The figure shows three views and two pictorial views of one solid part (mm, origin at its lowest corner). Answer the questions. A direction names the side the tool comes from. Coordinates: 2 decimals unless noted, no trailing zeros. Write each loop counter-clockwise with the first axis right and the second up, starting at its lowest first coordinate (ties: lowest second). Pieces come first, ordered by that corner, then holes. Notation, with made-up numbers: M 8.5,-3.5 L 18.5,-3.5 A7 cw 18.5,8.5 Z; hole C 79.5,72 d10. An arc over 180 degrees is marked long. Answer as CSV lines item,"result".
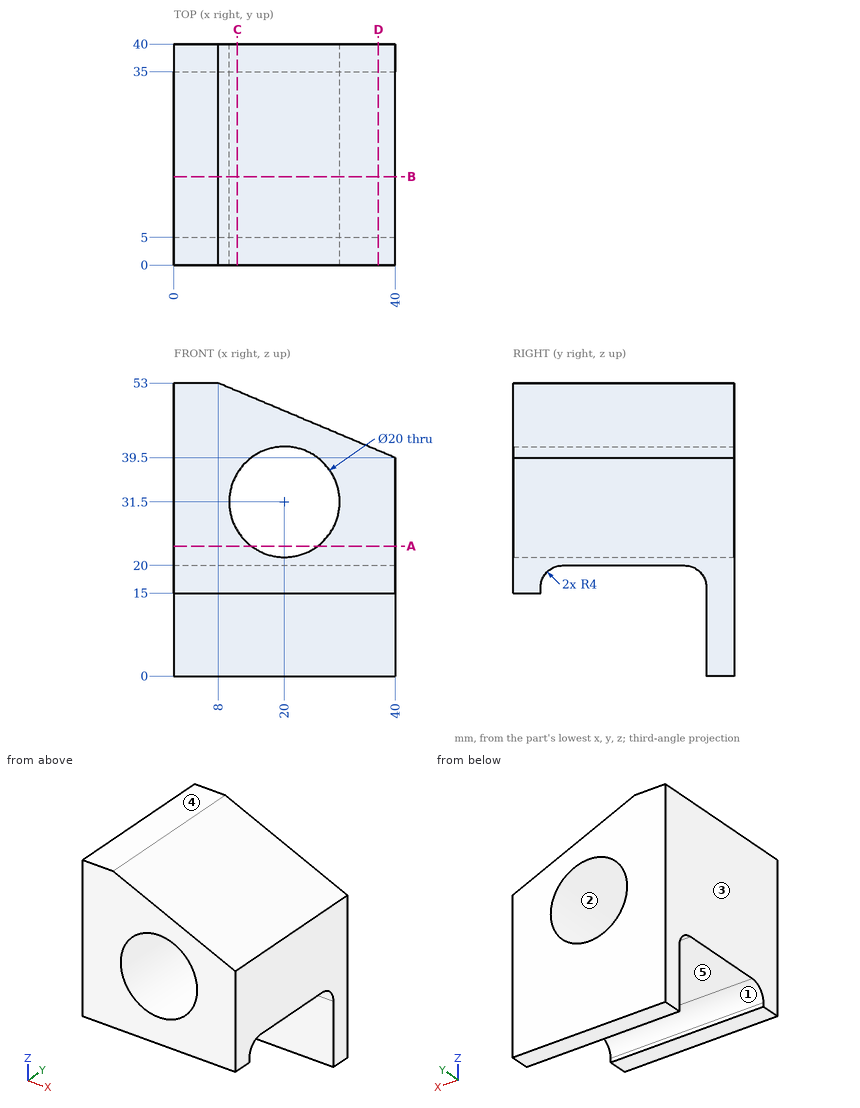
Q1. Flat-ended cylindrical pins translate along their axes: pin 1 Ø6 at (x, y) = (32, 19.5) entering from -Z; pin 2 Ø2.5 at (x, y) = (19, 3) entering from -Z; pin 3 Ø24 at (x, y) = (16.5, 21.5) entering from -Z. Find the tip coordinate at first contact, or state that the pin passes through.
Output:
pin 1,"z = 20"
pin 2,"z = 15"
pin 3,"z = 19.12"
Q2. Find section A-A (z = 23.5). Give the vertices of the cut face in (x, y).
Output:
outline,"M 0,0 L 14,0 L 14,40 L 0,40 Z; M 26,0 L 40,0 L 40,40 L 26,40 Z"
Q3. Find section D-D (x = 37). Give the vertices of the cut face in (y, z).
Output:
outline,"M 0,15 L 5,15 L 5,16 A4 cw 9,20 L 31,20 A4 cw 35,16 L 35,0 L 40,0 L 40,40.77 L 0,40.77 Z"
Q4. Find section B-B (y = 16). Give the vertices of the cut face in (x, z), and give its area (3 significant figures).
Output:
outline,"M 0,20 L 40,20 L 40,39.5 L 8,53 L 0,53 Z; hole C 20,31.5 d20"
area,"790 mm2"
Q5. The mould has two halves that part along Z. Classify the marked faces 1, 2 and 3: pulls with the +Z half, pulls with the -Z half, needs draft (parallel to the pull), parting line crosses it, or undercut.
Output:
face 1,"pulls with the -Z half"
face 2,"undercut"
face 3,"needs draft"
Q6. Find section C-C (x = 11.5). Give the vertices of the cut face in (y, z), and give its area (3 significant figures).
Output:
outline,"M 0,15 L 5,15 L 5,16 A4 cw 9,20 L 31,20 A4 cw 35,16 L 35,0 L 40,0 L 40,26.23 L 0,26.23 Z; M 0,36.77 L 40,36.77 L 40,51.52 L 0,51.52 Z"
area,"971 mm2"
Q7. For the marked faces 4 and 5, determine the directions among +Z, -Z, +X, -X, +Y, -Y from which every point of the face is accessible in a straight line to the end or side of a thin tool.
Output:
face 4,"+Z, +X, -X, +Y, -Y"
face 5,"-Z, +X, -X"
Q8. Straight lines are drawn through the part: line 1 (X direction, y = 28, z = 31); line 2 (Z direction, x = 20, y = 11.5); line 3 (Z direction, x = 6, y = 20.5). For each, find the intervals that lie inside material, in ascending order.
Output:
line 1,"0 to 10.01, 29.99 to 40"
line 2,"20 to 21.5, 41.5 to 47.94"
line 3,"20 to 53"
